Can you work these out from the model? Positions are in its coordinate system, mm. Give positions to 0.01 mm unless a question says otherwise; leave off trailing zeros. Order: outer loops, then holes, each group sorted by start corner. A loop starts at its lowest first (then second) coordinate and runs counter-clockwise, first axis right, second up.
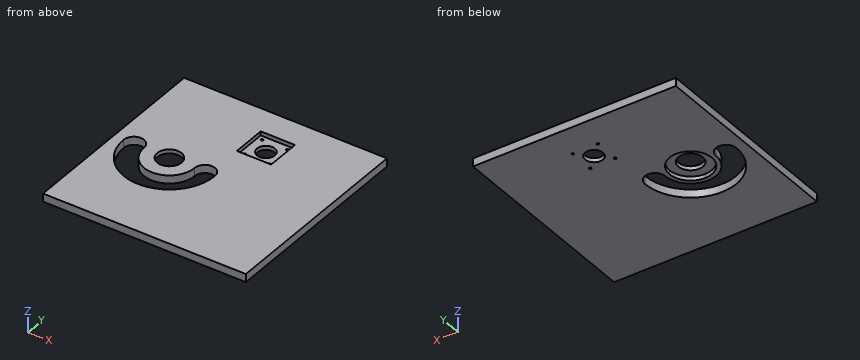
```python
from build123d import *

# Parameters (mm, degrees)
F0_W     = 250
F0_H     = 250
F0_R     = 15
F0_R_2   = 1.5
F0_R_3   = 11
F1_DEPTH = 10
F3_W     = 42.3
F3_H     = 42.3
F4_DEPTH = 5
F5_DEPTH = 5


with BuildPart() as f1:
    # F0 (on Top) → F1 (new body)
    with BuildSketch(Plane.XY):
        Rectangle(F0_W, F0_H)
        with BuildLine():
            ThreePointArc((0, 0), (-56.25, -56.25), (-112.5, 0))
            ThreePointArc((-112.5, 0), (-100, 12.5), (-87.5, 0))
            ThreePointArc((-87.5, 0), (-56.25, -31.25), (-25, 0))
            ThreePointArc((-25, 0), (-12.5, 12.5), (0, 0))
        make_face(mode=Mode.SUBTRACT)
        with Locations((-56.25, 0)):
            Circle(F0_R, mode=Mode.SUBTRACT)
        with Locations((-1.5696519672, 54.6803480328)):
            Circle(F0_R_2, mode=Mode.SUBTRACT)
        with Locations((-1.5696519672, 85.6803480328)):
            Circle(F0_R_2, mode=Mode.SUBTRACT)
        with Locations((29.4303480328, 54.6803480328)):
            Circle(F0_R_2, mode=Mode.SUBTRACT)
        with Locations((13.9303480328, 70.1803480328)):
            Circle(F0_R_3, mode=Mode.SUBTRACT)
        with Locations((29.4303480328, 85.6803480328)):
            Circle(F0_R_2, mode=Mode.SUBTRACT)
    extrude(amount=F1_DEPTH)

    # F3 (on face) → F4 (cut)
    with BuildSketch(Plane.XY.offset(10)):
        with Locations((13.9303480328, 70.1803480328)):
            Rectangle(F3_W, F3_H)
    extrude(amount=-F4_DEPTH, mode=Mode.SUBTRACT)

    # F2 (on face) → F5 (cut)
    with BuildSketch(Plane(origin=(0, 0, 0), x_dir=(1, 0, 0), z_dir=(0, 0, -1))):
        with BuildLine():
            ThreePointArc((-30.25, 0), (-37.8652236891, 18.3847763109), (-56.25, 26))
            ThreePointArc((-56.25, 26), (-74.6347763109, -18.3847763109), (-30.25, 0))
        make_face()
        with BuildLine():
            ThreePointArc((-41.25, 0), (-66.8566017178, -10.6066017178), (-56.25, 15))
            ThreePointArc((-56.25, 15), (-45.6433982822, 10.6066017178), (-41.25, 0))
        make_face(mode=Mode.SUBTRACT)
    extrude(amount=-F5_DEPTH, mode=Mode.SUBTRACT)


with BuildPart() as f6_1:
    # F6: copy of F1
    add(f1.part)


solid = f1.part
```
1) If I drill on line 1 (X direction, y = -1.5, z = 2); line 2 (Y direction, x = -56.25, z = 3.9); line 3 (Y direction, x = -55.5, z = 7.75) (3 decimals), over which ranges is the centre line in solid material (lowest first)?
2) Suppose I cut it at A-A (z = 7.75). Please give me the cut outline in (x, y).
3) Suppose I cut it at D-D (x = -100). Please give me the cut outline in (y, z), and give its area (3 significant figures).
4) Suppose I cut it at C-C (y = 64). Please give me the cut outline in (x, z).
5) I'm going to push flat-ended pins straight in: pin 1 Ø15.5 at (x, y) = (-61, -6) entering from -Z; pin 2 Ø4 at (x, y) = (29.43, 85.68) entering from +Z. Where does each tip first touch, or does it pass through?
6) Suppose I cut it at B-B (x = -65). Please give me the cut outline in (y, z), and give its area (3 significant figures).
Results:
1. line 1: x = -125 to -112.48, -87.46 to -82.21, -30.29 to -25.04, -0.02 to 125
1. line 2: y = -125 to -56.25, -31.25 to -26, 26 to 125
1. line 3: y = -125 to -56.245, -31.241 to -14.981, 14.981 to 125
2. outline: (-125, -125) - (125, -125) - (125, 125) - (-125, 125) - close; hole (-112.5, 0) arc R56.25 ccw to (0, 0) arc R12.5 ccw to (-25, 0) arc R31.25 cw to (-87.5, 0) arc R12.5 ccw to start; hole circle Ø30 at (-56.25, 0); hole (-7.22, 49.03) - (35.08, 49.03) - (35.08, 91.33) - (-7.22, 91.33) - close
3. outline: (-125, 0) - (-35.36, 0) - (-35.36, 10) - (-125, 10) - close; (12.5, 0) - (125, 0) - (125, 10) - (12.5, 10) - close
3. area: 2,020 mm2
4. outline: (-125, 0) - (4.83, 0) - (4.83, 5) - (-7.22, 5) - (-7.22, 10) - (-125, 10) - close; (23.03, 0) - (125, 0) - (125, 10) - (35.08, 10) - (35.08, 5) - (23.03, 5) - close
5. pin 1: stops at z = 5
5. pin 2: stops at z = 5
6. outline: (-125, 0) - (-55.57, 0) - (-55.57, 10) - (-125, 10) - close; (-30, 0) - (-24.48, 0) - (-24.48, 5) - (-12.18, 5) - (-12.18, 10) - (-30, 10) - close; (12.18, 5) - (24.48, 5) - (24.48, 0) - (125, 0) - (125, 10) - (12.18, 10) - close
6. area: 1,880 mm2
